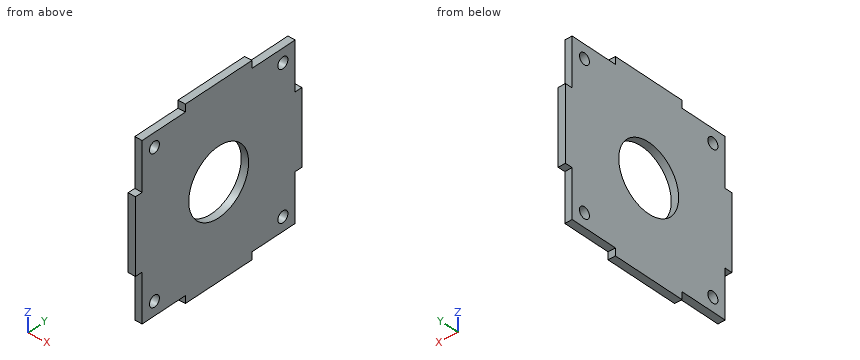
Autodesk Inventor part; units mm, degrees
ref_plane "YZ Plane" through (0, 0, 0) normal (1, 0, 0) x (0, 1, 0)
ref_plane "XZ Plane" through (0, 0, 0) normal (0, 1, 0) x (-1, 0, 0)
ref_plane "XY Plane" through (0, 0, 0) normal (0, 0, 1) x (1, 0, 0)
sketch "Sketch1" plane through (0, 0, 0) normal (1, 0, 0) x (0, 1, 0)
  line L0 (-25, -25) -> (25, -25)
  line L1 (25, -25) -> (25, 25)
  line L2 (25, 25) -> (-25, 25)
  line L3 (-25, 25) -> (-25, -25)
  line L4 (-25, -25) -> (25, 25) construction
  line L5 (25, -25) -> (-25, 25) construction
  line L6 (-24, -24) -> (24, -24)
  line L7 (24, -24) -> (24, 24)
  line L8 (24, 24) -> (-24, 24)
  line L9 (-24, 24) -> (-24, -24)
  line L10 (-24, -24) -> (24, 24) construction
  line L11 (24, -24) -> (-24, 24) construction
  point P0 (0, 0)
  dimension "d0" = 50
  dimension "d1" = 50
  dimension "d2" = 48
  dimension "d3" = 48
extrude "Extrusion1" add sketch "Sketch1" along normal blind 2 contours L3 L2 L1 L0 | L9 L8 L7 L6
sketch "Sketch3" plane through (0, 0, 0) normal (-1, 0, 0) x (0, 0, 1)
  line L0 (19.3, -19.3) -> (-19.3, -19.3)
  line L1 (-19.3, -19.3) -> (-19.3, 19.3)
  line L2 (-19.3, 19.3) -> (19.3, 19.3)
  line L3 (19.3, 19.3) -> (19.3, -19.3)
  line L4 (19.3, -19.3) -> (-19.3, 19.3) construction
  line L5 (-19.3, -19.3) -> (19.3, 19.3) construction
  circle A0 centre (-19.3, 19.3) radius 1.5
  circle A1 centre (19.3, 19.3) radius 1.5555
  circle A2 centre (19.3, -19.3) radius 1.5555
  circle A3 centre (-19.3, -19.3) radius 1.5555
  point P0 (0, 0)
  dimension "d6" = 38.6
  dimension "d7" = 38.6
  dimension "d8" = 3
  dimension "d9" = 3.111
  dimension "d10" = 3.111
  dimension "d11" = 3.111
hole "Hole1" at (0, 19.3, -19.3) direction (1, 0, 0) diameter 3 end through all
sketch "Sketch4" plane through (0, 0, 0) normal (-1, 0, 0) x (0, 0, 1)
  line L0 (-19.3, -19.3) -> (19.3, -19.3)
  line L1 (19.3, -19.3) -> (19.3, 19.3)
  line L2 (19.3, 19.3) -> (-19.3, 19.3)
  line L3 (-19.3, 19.3) -> (-19.3, -19.3)
  line L4 (-19.3, -19.3) -> (19.3, 19.3) construction
  line L5 (19.3, -19.3) -> (-19.3, 19.3) construction
  circle A0 centre (19.3, 19.3) radius 1.5
  point P0 (0, 0)
  dimension "d19" = 38.6
  dimension "d20" = 38.6
  dimension "d21" = 3
hole "Hole2" at (0, 19.3, 19.3) direction (1, 0, 0) diameter 3 end through all
sketch "Sketch5" plane through (0, 0, 0) normal (-1, 0, 0) x (0, 0, 1)
  line L0 (19.3, -19.3) -> (-19.3, -19.3)
  line L1 (-19.3, -19.3) -> (-19.3, 19.3)
  line L2 (-19.3, 19.3) -> (19.3, 19.3)
  line L3 (19.3, 19.3) -> (19.3, -19.3)
  line L4 (19.3, -19.3) -> (-19.3, 19.3) construction
  line L5 (-19.3, -19.3) -> (19.3, 19.3) construction
  circle A0 centre (-19.3, -19.3) radius 1.5
  point P0 (0, 0)
  dimension "d29" = 38.6
  dimension "d30" = 38.6
  dimension "d31" = 3
hole "Hole3" at (0, -19.3, -19.3) direction (1, 0, 0) diameter 3 end through all
sketch "Sketch6" plane through (0, 0, 0) normal (-1, 0, 0) x (0, 0, 1)
  line L0 (19.3, -19.3) -> (-19.3, -19.3)
  line L1 (-19.3, -19.3) -> (-19.3, 19.3)
  line L2 (-19.3, 19.3) -> (19.3, 19.3)
  line L3 (19.3, 19.3) -> (19.3, -19.3)
  line L4 (19.3, -19.3) -> (-19.3, 19.3) construction
  line L5 (-19.3, -19.3) -> (19.3, 19.3) construction
  circle A0 centre (19.3, -19.3) radius 1.5
  point P0 (0, 0)
  dimension "d39" = 38.6
  dimension "d40" = 38.6
  dimension "d41" = 3
hole "Hole4" at (0, -19.3, 19.3) direction (1, 0, 0) diameter 3 end through all
sketch "Sketch7" plane through (0, 0, 0) normal (-1, 0, 0) x (0, 0, 1)
  line L0 (23, -23) -> (-23, -23)
  line L1 (-23, -23) -> (-23, 23)
  line L2 (-23, 23) -> (23, 23)
  line L3 (23, 23) -> (23, -23)
  line L4 (23, -23) -> (-23, 23) construction
  line L5 (-23, -23) -> (23, 23) construction
  line L6 (-25, 25) -> (25, 25)
  line L7 (10, 21) -> (-10, 21)
  line L8 (-10, 21) -> (-10, 25)
  line L9 (-10, 25) -> (10, 25)
  line L10 (10, 25) -> (10, 21)
  line L11 (10, 21) -> (-10, 25) construction
  line L12 (-10, 21) -> (10, 25) construction
  line L13 (21, -10) -> (25, -10)
  line L14 (25, -10) -> (25, 10)
  line L15 (25, 10) -> (21, 10)
  line L16 (21, 10) -> (21, -10)
  line L17 (21, -10) -> (25, 10) construction
  line L18 (25, -10) -> (21, 10) construction
  line L19 (25, -25) -> (-25, -25)
  line L20 (-10, -21) -> (10, -21)
  line L21 (10, -21) -> (10, -25)
  line L22 (10, -25) -> (-10, -25)
  line L23 (-10, -25) -> (-10, -21)
  line L24 (-10, -21) -> (10, -25) construction
  line L25 (10, -21) -> (-10, -25) construction
  line L26 (-25.0252, 10) -> (-20.9748, 10)
  line L27 (-20.9748, 10) -> (-20.9748, -10)
  line L28 (-20.9748, -10) -> (-25.0252, -10)
  line L29 (-25.0252, -10) -> (-25.0252, 10)
  line L30 (-25.0252, 10) -> (-20.9748, -10) construction
  line L31 (-20.9748, 10) -> (-25.0252, -10) construction
  line L32 (25, -25) -> (-25, -25)
  line L33 (-25, -25) -> (-25, 25)
  line L34 (-25, 25) -> (25, 25)
  line L35 (25, 25) -> (25, -25)
  line L36 (25, -25) -> (-25, 25) construction
  line L37 (-25, -25) -> (25, 25) construction
  point P0 (0, 0)
  point P1 (0, 23)
  point P2 (23, 0)
  point P3 (0, -23)
  point P4 (-23, 0)
  point P5 (-10, 23)
  point P6 (10, 23)
  point P7 (23, 10)
  point P8 (23, -10)
  point P9 (10, -23)
  point P10 (-10, -23)
  point P11 (-23, -10)
  point P12 (-23, 10)
  point P13 (10, 25)
  point P14 (-25, 10)
  point P15 (-25, -10)
  point P16 (-10, -25)
  dimension "d49" = 46
  dimension "d50" = 46
  dimension "d51" = 20
  dimension "d52" = 20
  dimension "d53" = 20
  dimension "d54" = 20
extrude "Extrusion3" cut sketch "Sketch7" against normal blind 2 contours L3 L13 L35 L19 L21 L0 | L23 L19 L33 L28 L1 L0 | L3 L2 L10 L6 L35 L15 | L26 L33 L6 L8 L2 L1
sketch "Sketch8" plane through (2, 0, 0) normal (1, 0, 0) x (0, 0, -1)
  circle A0 centre (0, 0) radius 9
  dimension "d59" = 18
extrude "Extrusion4" cut sketch "Sketch8" against normal blind 2
sketch "Sketch9" plane through (2, 0, 0) normal (1, 0, 0) x (0, 0, -1)
  line L0 (13.75, -13.75) -> (-13.75, -13.75)
  line L1 (-13.75, -13.75) -> (-13.75, 13.75)
  line L2 (-13.75, 13.75) -> (13.75, 13.75)
  line L3 (13.75, 13.75) -> (13.75, -13.75)
  line L4 (13.75, -13.75) -> (-13.75, 13.75) construction
  line L5 (-13.75, -13.75) -> (13.75, 13.75) construction
  circle A0 centre (-13.75, 13.75) radius 1
  circle A1 centre (13.75, 13.75) radius 1
  circle A2 centre (13.75, -13.75) radius 1
  circle A3 centre (-13.75, -13.75) radius 1
  point P0 (0, 0)
  dimension "d62" = 27.5
  dimension "d63" = 27.5
  dimension "d64" = 2
  dimension "d65" = 2
  dimension "d66" = 2
  dimension "d67" = 2
extrude "Extrusion5" [suppressed]
properties part number "UpperSide" material "Aluminum 6061, Welded"
The model under review builds one solid part; all positions refer to its coordinate system, in mm. Give positions to 0.01 mm unless a question says otherwise; leave off trailing zeros. Write each loop counter-clockwise with the first axis right and the second up, starting at its lowest first coordinate (ties: lowest second). Pieces come first, ordered by that corner, then holes.
1. Add section A-A, the plane z = 0. Write out the cut boundary in (x, y).
2. Wall thickness on L1, parallel to Y at x = 0.85, z = -19.3; L2, parallel to Y at x = 1, z = -0.5: over which ranges is each line inside the solid? List them lowest first.
3. For P1, Ø1, axis at x = 1.5, y = 15.5, coming from the -Z side; P2, Ø0.6, axis at x = 1.5, z = 24, coming from the +Y side; P3, Ø1, axis at x = 0.5, y = 15.5, coming from the +Z side; P4, Ø1.8, axis at y = -19.3, z = 19.3, coming from the -X side, all flat-tipped, find the tip position at first contact; note any pin that passes through.
4. Add section B-B, the plane y = 19.3. Write out the cut boundary in (x, z).
5. Add section D-D, the plane x = 1.1. Write out the cut boundary in (y, z), plus the area to 3 significant figures.
Worked answers:
1. outline: (0, -25) - (2, -25) - (2, -9) - (0, -9) - close; (0, 9) - (2, 9) - (2, 25) - (0, 25) - close
2. L1: y = -23 to -20.8, -17.8 to 17.8, 20.8 to 23
2. L2: y = -25 to -8.99, 8.99 to 25
3. P1: stops at z = -23
3. P2: stops at y = 10
3. P3: stops at z = 23
3. P4: passes through
4. outline: (0, -23) - (2, -23) - (2, -20.8) - (0, -20.8) - close; (0, -17.8) - (2, -17.8) - (2, 17.8) - (0, 17.8) - close; (0, 20.8) - (2, 20.8) - (2, 23) - (0, 23) - close
5. outline: (-25, -10) - (-23, -10) - (-23, -23) - (-10, -23) - (-10, -25) - (10, -25) - (10, -23) - (23, -23) - (23, -10) - (25, -10) - (25, 10) - (23, 10) - (23, 23) - (10, 23) - (10, 25) - (-10, 25) - (-10, 23) - (-23, 23) - (-23, 10) - (-25, 10) - close; hole circle Ø3 at (-19.3, -19.3); hole circle Ø3 at (-19.3, 19.3); hole circle Ø18 at (0, 0); hole circle Ø3 at (19.3, -19.3); hole circle Ø3 at (19.3, 19.3)
5. area: 1,990 mm2
